Input: part model. Units: mm. Frame: model coordinates. A direction names the side the tool comes from. Coordinates: 2 decimals unless noted, no trailing zeros. Order: outer loops, then holes, each group sorted by start corner. A loop starts at its lowest first (then second) coordinate and runs counter-clockwise, first axis right, second up. Notation, with made-up numbers: (59.5, -24) -> (106.5, -24) arc R21 ccw to (106.5, 11) -> close; hole circle Ø1 at (20.5, 16). An arc over 180 degrees is marked (long way). Answer as CSV lines item,"result".
from build123d import *

# Parameters (mm, degrees)
ESQUISSE1_W          = 60
ESQUISSE1_H          = 60
BASE_EXTRUSION_DEPTH = 7
CONG_2_R             = 2
ESQUISSE14_R         = 11.25
BOSS_EXTRU_12_DEPTH  = 20


with BuildPart() as part:
    # Esquisse1 → Base-Extrusion (new body)
    with BuildSketch(Plane.XY):
        Rectangle(ESQUISSE1_W, ESQUISSE1_H)
    extrude(amount=BASE_EXTRUSION_DEPTH)

    # Congé2
    cong_2_edges = [part.edges().sort_by_distance(p)[0] for p in [
        (-30, 30, 3.5),
        (30, 30, 3.5),
        (30, -30, 3.5),
        (-30, -30, 3.5),
    ]]
    fillet(cong_2_edges, radius=CONG_2_R)

    # Esquisse14 → Boss.-Extru.12 (add)
    with BuildSketch(Plane(origin=(0, 0, 0), x_dir=(-1, 0, 0), z_dir=(0, 0, -1))):
        with Locations(Location((0, 0, 0), (0, 0, 180))):
            Circle(ESQUISSE14_R)
    extrude(amount=BOSS_EXTRU_12_DEPTH)


solid = part.part
1. Reachability of faces 1 (the face through (-14, 0, 0)), 2 (the face through (29.43, 29.4, 3.55)) from +Z, -Z, +X, -X, +Y, -Y: full face, straight path, thin tool, end or side. Return the list, or none.
Findings:
face 1,"-Z"
face 2,"+Z, -Z, +X, +Y"
2. Ray query, line 1 along Z through (x, y) = (0, -25); line 2 along X through (y, z) = (5, -7.25); line 3 along X through (y, z) = (1.5, -3.5). Return the intervals inside material, ascending.
Findings:
line 1,"z = 0 to 7"
line 2,"x = -10.08 to 10.08"
line 3,"x = -11.15 to 11.15"
3. Cut plane D-D (x = 15). Return the cut outline in (y, z), plus the area to 3 significant figures.
Findings:
outline,"(-30, 0) -> (30, 0) -> (30, 7) -> (-30, 7) -> close"
area,"420 mm2"
4. Cut plane C-C (z = -14.75). Return the cut outline in (x, y), plus the area to 3 significant figures.
Findings:
outline,"circle Ø22.5 at (0, 0)"
area,"398 mm2"
5. Contact query for flat-ended pins moving along their axis: pin 1 (1 mm diameter, centred on x = -17, y = -12, fed in from -Z); pin 2 (12 mm diameter, centred on y = -11.5, z = -8, fed in from -X); pin 3 (1 mm diameter, centred on y = 9.5, z = -8, fed in from +X). Output: stop coordinate, or through.
Findings:
pin 1,"stops at z = 0"
pin 2,"stops at x = -9.81"
pin 3,"stops at x = 6.75"
6. Cut plane A-A (x = 0). Return the cut outline in (y, z), plus the area to 3 significant figures.
Findings:
outline,"(-30, 0) -> (-11.25, 0) -> (-11.25, -20) -> (11.25, -20) -> (11.25, 0) -> (30, 0) -> (30, 7) -> (-30, 7) -> close"
area,"870 mm2"
